```python
from build123d import *

# Parameters (mm, degrees)
F0_R     = 10.15
F0_R_2   = 8.15
F1_DEPTH = 4
F2_R     = 12.15
F2_R_2   = 8.15
F3_DEPTH = 8
F4_W     = 7
F4_H     = 15
F5_DEPTH = 17.272
F6_W     = 9.9999997467
F6_H     = 4
F7_DEPTH = 3


with BuildPart() as f1:
    # F0 (on Top) → F1 (new body)
    with BuildSketch(Plane.XY):
        Circle(F0_R)
        Circle(F0_R_2, mode=Mode.SUBTRACT)
    extrude(amount=F1_DEPTH)

    # F2 (on face) → F3 (join)
    with BuildSketch(Plane(origin=(0, 0, 0), x_dir=(1, 0, 0), z_dir=(0, 0, -1))):
        Circle(F2_R)
        Circle(F2_R_2, mode=Mode.SUBTRACT)
    extrude(amount=F3_DEPTH)

    # F4 (on face) → F5 (cut)
    with BuildSketch(Plane(origin=(0, 0, -8), x_dir=(1, 0, 0), z_dir=(0, 0, -1))):
        with Locations((-0.0862163142, 0.1069762555)):
            Rectangle(F4_W, F4_H)
    extrude(amount=-F5_DEPTH, mode=Mode.SUBTRACT)

    # F6 (on face) → F7 (join)
    with BuildSketch(Plane(origin=(0, 0, -8), x_dir=(1, 0, 0), z_dir=(0, 0, -1))):
        with BuildLine():
            ThreePointArc((-3.5862161876, 7.3185760583), (-8.1500001267, 0), (-3.5862161876, -7.3185760583))
            Line((-3.5862161876, -7.3185760583), (-3.5862161876, -7.3930236179))
            Line((-3.5862161876, -7.3930236179), (-3.4301165755, -7.3930236179))
            ThreePointArc((-3.4301165755, -7.3930236179), (-0.0089980782, -8.1499949061), (3.4137835591, -7.4005796899))
            Line((3.4137835591, -7.4005796899), (3.4137835591, -7.3930236179))
            Line((3.4137835591, -7.3930236179), (3.4301165755, -7.3930236179))
            ThreePointArc((3.4301165755, -7.3930236179), (8.1499949061, 0.0089980782), (3.4137835591, 7.4005796899))
            Line((3.4137835591, 7.4005796899), (3.4137835591, 7.6069761288))
            Line((3.4137835591, 7.6069761288), (2.9251345458, 7.6069761288))
            ThreePointArc((2.9251345458, 7.6069761288), (0, 8.1499998733), (-2.9251345458, 7.6069761288))
            Line((-2.9251345458, 7.6069761288), (-3.5862161876, 7.6069761288))
            Line((-3.5862161876, 7.6069761288), (-3.5862161876, 7.3185760583))
        make_face()
        with Locations((-0.0862163142, -3.5)):
            Rectangle(F6_W, F6_H, mode=Mode.SUBTRACT)
        with Locations((-0.0862163142, 3.5)):
            Rectangle(F6_W, F6_H, mode=Mode.SUBTRACT)
        with BuildLine():
            Line((3.4137835591, -7.3930236179), (3.4137835591, -7.4005796899))
            ThreePointArc((3.4137835591, -7.4005796899), (3.4219521529, -7.396806162), (3.4301165755, -7.3930236179))
            Line((3.4301165755, -7.3930236179), (3.4137835591, -7.3930236179))
        make_face()
    extrude(amount=-F7_DEPTH)


solid = f1.part
```
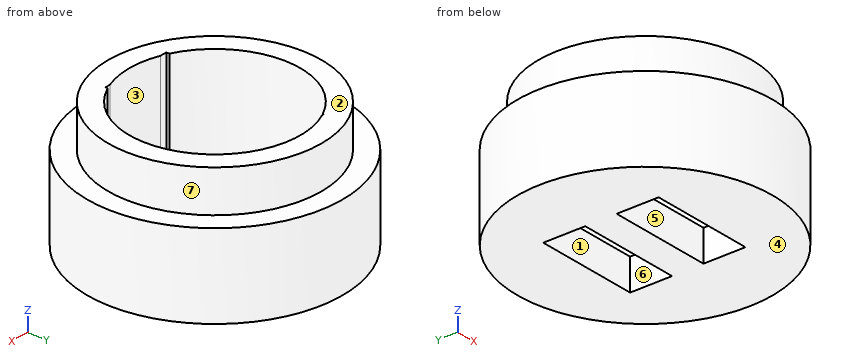
Could you check a few things on this model? Use its own coordinates, in mm. Face numbers are marked on the shaded views. A direction names the side the tool comes from. Round coordinates to 2 decimals unless told otherwise and drop trailing zeros. Loops run counter-clockwise (first coordinate to the right, second up) from the corner with the lowest first, then second, coordinate; pieces in that order, holes last. Notation, with made-up numbers: M -2.5,5 L 35.5,5 A20 cw 35.5,12 Z; hole C 77.25,72 d4. An arc over 180 degrees is marked long. Answer as CSV lines item,"result".
1) Imagine slicing it at B-B on z = -6. List the corners of the cut face in (x, y) for me, and give its area (3 significant figures).
From the geometry:
outline,"C 0,0 d24.3; hole M -5.09,-5.5 L 4.91,-5.5 L 4.91,-1.5 L -5.09,-1.5 Z; hole M -5.09,1.5 L 4.91,1.5 L 4.91,5.5 L -5.09,5.5 Z"
area,"384 mm^2"
2) For pin 1 Ø1.5 at (x, z) = (1, -7) entering from -Y; pin 2 Ø6 at (y, z) = (3.5, -7) entering from -X; pin 3 Ø3.5 at (y, z) = (-4, -6) entering from -X, each with a flat end and sliding along its axis, tell me the tip position at first contact or that it passes through.
From the geometry:
pin 1,"y = -12.15"
pin 2,"x = -12.14"
pin 3,"x = -11.94"
3) Imagine slicing it at A-A on x = 0. List the corners of the cut face in (y, z) for me.
From the geometry:
outline,"M -12.15,-8 L -5.5,-8 L -5.5,-5 L -8.15,-5 L -8.15,4 L -10.15,4 L -10.15,0 L -12.15,0 Z; M -1.5,-8 L 1.5,-8 L 1.5,-5 L -1.5,-5 Z; M 5.5,-8 L 12.15,-8 L 12.15,0 L 10.15,0 L 10.15,4 L 8.15,4 L 8.15,-5 L 5.5,-5 Z"
4) We'd pull the mould along Y, two halves only. Please class the marked faces 4, 5, 6 and 7: released by +Y, released by -Y, zero draft, split by the parting line, or undercut.
From the geometry:
face 4,"zero draft"
face 5,"undercut"
face 6,"undercut"
face 7,"split by the parting line"
5) Which directions (+Z, -Z, +X, -X, +Y, -Y) give clear straight access to the entire face, cutting with the end or side of a thin tool? Please do the marked faces 1, 2 and 3.
From the geometry:
face 1,"+Z, -Z"
face 2,"+Z, +X, -X, +Y, -Y"
face 3,"+Z"
6) Imagine slicing it at D-D on y = 0. List the corners of the cut face in (x, z) for me.
From the geometry:
outline,"M -12.15,-8 L 12.15,-8 L 12.15,0 L 10.15,0 L 10.15,4 L 8.15,4 L 8.15,-5 L -8.15,-5 L -8.15,4 L -10.15,4 L -10.15,0 L -12.15,0 Z"
7) If I drill on probe 1 along Z at (x, y) = (1.75, 1); probe 2 along Y at (x, z) = (-4, -2); probe 3 along X at (y, z) = (0, -2), over which ranges is the centre line in solid material (lowest first)?
From the geometry:
probe 1,"-8 to -5"
probe 2,"-11.47 to -7.1, 7.1 to 11.47"
probe 3,"-12.15 to -8.15, 8.15 to 12.15"
